The listing builds one solid part. Answer for the finished solid, in the listing's coordinates (mm). A direction names the side the tool comes from. Round coordinates to 2 decimals unless told otherwise and drop trailing zeros. Write each loop counter-clockwise with the first axis right and the second up, starting at its lowest first coordinate (ties: lowest second). Pieces come first, ordered by that corner, then holes. Notation, with made-up numbers: (9, 83.5) -> (21, 83.5) arc R20 ccw to (21, 118.5) -> close; hole circle Ø3 at (6, 14). An arc over 180 degrees is marked (long way). Write each question's results on one line, items separated by ' | '. Start each with the question number.
Autodesk Fusion 360 part; units mm, degrees
sketch "Sketch1" plane through (0, 0, 0) normal (0, 0, 1) x (1, 0, 0)
  line L0 (20, 63.2) -> (98, 63.2)
  line L1 (98, 63.2) -> (98, 20)
  line L2 (98, 20) -> (20, 20)
  line L3 (20, 20) -> (20, 63.2)
  dimension "d1" = 78
  dimension "d2" = 20
  dimension "d4" = 43.2
  dimension "d5" = 20
extrude "Extrude4" add sketch "Sketch1" along normal blind 6.6
sketch "Profondeurboite" plane through (0, 0, 6.6) normal (0, 0, 1) x (-1, 0, 0)
  line L0 (-20, -20) -> (-98, -20)
  line L1 (-98, -20) -> (-98, -63.2)
  line L2 (-98, -63.2) -> (-20, -63.2)
  line L3 (-20, -63.2) -> (-20, -20)
  line L4 (-97.2, -20.8) -> (-20.8, -20.8)
  line L5 (-20.8, -20.8) -> (-20.8, -62.4)
  line L6 (-20.8, -62.4) -> (-97.2, -62.4)
  line L7 (-97.2, -62.4) -> (-97.2, -20.8)
  dimension "d20" = 76.4
  dimension "d21" = 41.6
  dimension "d22" = 0.8
  dimension "d23" = 0.8
extrude "Extrude6" cut sketch "Profondeurboite" against normal blind 3.6 contours L4 L5 L6 L7
sketch "trous pour ecrous" plane through (0, 0, 0) normal (0, 0, 1) x (1, 0, 0)
  line L0 (20, 20) -> (20, 63.2)
  line L1 (20, 63.2) -> (98, 63.2)
  line L2 (98, 20) -> (20, 20)
  line L3 (98, 63.2) -> (98, 20)
  line L4 (26.0877, 55.85) -> (27.6754, 58.6)
  line L5 (27.6754, 58.6) -> (26.0877, 61.35)
  line L6 (26.0877, 61.35) -> (22.9123, 61.35)
  line L7 (22.9123, 61.35) -> (21.3246, 58.6)
  line L8 (21.3246, 58.6) -> (22.9123, 55.85)
  line L9 (22.9123, 55.85) -> (26.0877, 55.85)
  line L10 (95.0877, 21.85) -> (96.6754, 24.6)
  line L11 (96.6754, 24.6) -> (95.0877, 27.35)
  line L12 (95.0877, 27.35) -> (91.9123, 27.35)
  line L13 (91.9123, 27.35) -> (90.3246, 24.6)
  line L14 (90.3246, 24.6) -> (91.9123, 21.85)
  line L15 (91.9123, 21.85) -> (95.0877, 21.85)
  circle A0 centre (24.5, 58.6) radius 1.6
  circle A1 centre (93.5, 24.6) radius 1.6
  point P0 (24.5, 58.6)
  point P1 (93.5, 24.6)
  dimension "d32" = 2.75
  dimension "d33" = 4.5
  dimension "d34" = 4.6
  dimension "d35" = 2.75
  dimension "d36" = 4.6
  dimension "d37" = 4.5
  dimension "d38" = 3.2
  dimension "d39" = 3.2
extrude "Extrude7" cut sketch "trous pour ecrous" along normal blind 3 contours A0 | A1
extrude "Extrude8" cut sketch "trous pour ecrous" along normal blind 2.7 contours L4 L5 L6 L7 L8 L9 | L10 L11 L12 L13 L14 L15
sketch "Extensions decrous" plane through (0, 0, 3) normal (0, 0, 1) x (-1, 0, 0)
  circle A0 centre (-24.5, -58.6) radius 1.6
  circle A1 centre (-93.5, -24.6) radius 1.6
  line L0 (-97.2, -62.4) -> (-20.8, -62.4)
  line L1 (-20.8, -62.4) -> (-20.8, -20.8)
  line L2 (-20.8, -20.8) -> (-97.2, -20.8)
  line L3 (-97.2, -20.8) -> (-97.2, -62.4)
  circle A2 centre (-24.5, -58.6) radius 3.9
  circle A3 centre (-93.5, -24.6) radius 3.9
  circle A4 centre (-93.5, -58.6) radius 3.9
  line L4 (-24.5, -58.6) -> (-97.2, -58.6)
  line L5 (-20, -63.2) -> (-98, -63.2)
  line L6 (-93.5, -24.6) -> (-93.5, -62.4)
  line L7 (-24.5, -58.6) -> (-24.5, -20.8)
  line L8 (-93.5, -24.6) -> (-20.8, -24.6)
  line L9 (-98, -20) -> (-20, -20)
  line L10 (-20, -20) -> (-20, -63.2)
  circle A5 centre (-24.5, -24.6) radius 3.9
  point P0 (-24.5, -58.6)
  point P1 (-93.5, -24.6)
  dimension "d44" = 7.8
  dimension "d45" = 7.8
  dimension "d48" = 7.8
  dimension "d49" = 7.8
extrude "Extrude9" add sketch "Extensions decrous" along normal blind 2 contours A0 L0 L1 A2 L4 L7 | A0 A2 L4 L7 | A1 L2 L3 A3 L6 L8 | A1 A3 L6 L8
extrude "Extrude10" add sketch "Extensions decrous" along normal blind 2 contours L7 L8 A5 | L1 L7 L8 A5 | A4 L4 L6 | L0 A4 L4 L6 | L2 L7 L8 A5 | L1 L2 L7 L8 A5 | L3 A4 L4 L6 | L0 L3 A4 L4 L6
sketch "planDroite" plane through (0, 0, 2.7) normal (0, 0, -1) x (1, 0, 0)
  circle A0 centre (93.5, -24.6) radius 1.6
  line L0 (95.0877, -21.85) -> (91.9123, -21.85)
  line L1 (91.9123, -21.85) -> (90.3246, -24.6)
  line L2 (90.3246, -24.6) -> (91.9123, -27.35)
  line L3 (91.9123, -27.35) -> (95.0877, -27.35)
  line L4 (95.0877, -27.35) -> (96.6754, -24.6)
  line L5 (96.6754, -24.6) -> (95.0877, -21.85)
  line L6 (95.0877, -21.85) -> (95.0877, -27.35)
  line L7 (91.9123, -21.85) -> (91.9123, -27.35)
  line L8 (91.9123, -26.2) -> (95.0877, -26.2)
  line L9 (95.0877, -23) -> (91.9123, -23)
sketch "PlanGauche" plane through (0, 0, 2.7) normal (0, 0, -1) x (1, 0, 0)
  circle A0 centre (24.5, -58.6) radius 1.6
  line L0 (26.0877, -55.85) -> (22.9123, -55.85)
  line L1 (22.9123, -55.85) -> (21.3246, -58.6)
  line L2 (21.3246, -58.6) -> (22.9123, -61.35)
  line L3 (22.9123, -61.35) -> (26.0877, -61.35)
  line L4 (26.0877, -61.35) -> (27.6754, -58.6)
  line L5 (27.6754, -58.6) -> (26.0877, -55.85)
  line L6 (22.9123, -55.85) -> (22.9123, -61.35)
  line L7 (26.0877, -61.35) -> (26.0877, -55.85)
  line L8 (26.0877, -57) -> (22.9123, -57)
  line L9 (26.0877, -60.2) -> (22.9123, -60.2)
extrude "Extrude11" cut sketch "planDroite" sketch "PlanGauche" against normal blind 0.6 contours A0 L6 L9 | A0 L6 L8 | A0 L7 L9 | A0 L7 L8 of sketch 2 contours A0 L7 L8 | A0 L7 L9 | A0 L6 L8 | A0 L6 L9
extrude "Extrude12" cut sketch "planDroite" sketch "PlanGauche" against normal blind 0.3 contours L0 L6 L7 L9 | L3 L6 L7 L8 of sketch 2 contours L0 L6 L7 L8 | L3 L6 L7 L9
extrude "Extrude13" add 4 faces at (48.6758, 46.7122, 3) (48.6758, 46.7122, 3) (21.5219, 61.785, 3) (48.6758, 46.7122, 3) along direction (0, 0, 1) up to surface end surface through (0, 0, 5) normal (0, 0, 1) offset 0
extrude "Extrude14" add 4 faces at (47.1385, 34.5234, 5) (47.1385, 34.5234, 5) (47.1385, 34.5234, 5) (47.1385, 34.5234, 5) along direction (0, 0, 1) blind 0.1
Q1. For faces 4 (the flat face through (21, 22, 3)), 5 (the flat face through (92.2, 25.9, 3.3)), determine the directions among +Z, -Z, +X, -X, +Y, -Y from which every point of the face is accessible in a straight line to the end or side of a thin tool.
Q2. Find the intervals of material crossed by line 1 (X direction, y = 24.6, z = 4.25); line 2 (Y direction, x = 44, z = 6); line 3 (Y direction, x = 93.5, z = 3.8), in increasing order.
Q3. Each of these flat-tipped pins is pushed along its axis until it touches: pin 1 (0.6 mm diameter, centred on x = 92.5, y = 26.5, fed in from -Z); pin 2 (2 mm diameter, centred on x = 22, y = 22, fed in from +Z); pin 3 (0.5 mm diameter, centred on x = 96, y = 24, fed in from -Z). Where does it stop, or does it pass through?
Q4. Determine the mould class of faces 1 (the flat face through (98, 42, 3)), 2 (the flat face through (58, 63.2, 3)), 3 (the flat face through (58, 62.4, 6)) for opening direction X: pulls with the +X half, pulls with the -X half, needs draft (parallel to the pull), parting line crosses it, or undercut.
Q5. The part is cut by section A-A, the plane x = 33.5. Write down the section's boundary in (y, z), then the cut area to 3 significant figures.
Q6. The part is cut by section B-B, the plane y = 40. Write down the section's boundary in (x, z), then the cut area to 3 significant figures.
Answers follow:
1) face 4: +Z | face 5: -Z
2) line 1: 20 to 91.9, 95.1 to 98 | line 2: 20 to 20.8, 62.4 to 63.2 | line 3: 20 to 23, 26.2 to 63.2
3) pin 1: z = 3 | pin 2: z = 5.1 | pin 3: z = 2.7
4) face 1: pulls with the +X half | face 2: needs draft | face 3: undercut
5) outline: (20, 0) -> (63.2, 0) -> (63.2, 6.6) -> (62.4, 6.6) -> (62.4, 5.1) -> (20.8, 5.1) -> (20.8, 6.6) -> (20, 6.6) -> close | area: 223 mm^2
6) outline: (20, 0) -> (98, 0) -> (98, 6.6) -> (97.2, 6.6) -> (97.2, 5.1) -> (20.8, 5.1) -> (20.8, 6.6) -> (20, 6.6) -> close | area: 400 mm^2
